```python
from build123d import *

# Parameters (mm, degrees)
SKETCH1_R                = 12.7
BOSS_EXTRUDE1_DEPTH      = 4.7752
SKETCH2_R                = 5.334
BOSS_EXTRUDE2_DEPTH      = 24.13
SKETCH3_R                = 1.27
BOSS_EXTRUDE3_DEPTH      = 2.54
BOSS_EXTRUDE3_DEPTH_BACK = 17.78
SKETCH6_W                = 2.54
SKETCH6_H                = 1.27
BOSS_EXTRUDE4_DEPTH      = 2.54


with BuildPart() as part:
    # Sketch1 → Boss-Extrude1 (new body)
    with BuildSketch(Plane.XY):
        Circle(SKETCH1_R)
    extrude(amount=BOSS_EXTRUDE1_DEPTH)

    # Sketch2 → Boss-Extrude2 (add)
    with BuildSketch(Plane(origin=(0, 0, 0), x_dir=(-1, 0, 0), z_dir=(0, 0, -1))):
        Circle(SKETCH2_R)
    extrude(amount=BOSS_EXTRUDE2_DEPTH)

    # Sketch3 → Boss-Extrude3 (add, two sides)
    with BuildSketch(Plane.XY.offset(4.7752)) as boss_extrude3_sk:
        with Locations((0, 9.525)):
            Circle(SKETCH3_R)
        with Locations((8.248891971, 4.7625)):
            Circle(SKETCH3_R)
        with Locations((8.248891971, -4.7625)):
            Circle(SKETCH3_R)
        with Locations((0, -9.525)):
            Circle(SKETCH3_R)
        with Locations((-8.248891971, -4.7625)):
            Circle(SKETCH3_R)
        with Locations((-8.248891971, 4.7625)):
            Circle(SKETCH3_R)
    extrude(amount=BOSS_EXTRUDE3_DEPTH)
    extrude(boss_extrude3_sk.sketch, amount=-BOSS_EXTRUDE3_DEPTH_BACK)

    # Sketch6 → Boss-Extrude4 (add)
    with BuildSketch(Plane(origin=(0, 0, 0), x_dir=(-1, 0, 0), z_dir=(0, 0, -1))):
        Polygon((1.482073869, 3.837027241), (2.581926131, 3.202027241), (3.851926131, 5.401731767), (2.752073869, 6.036731767), align=None)
        with Locations((5.334, 0)):
            Rectangle(SKETCH6_W, SKETCH6_H)
        Polygon((2.581926131, -3.202027241), (3.851926131, -5.401731767), (2.752073869, -6.036731767), (1.482073869, -3.837027241), align=None)
        Polygon((-1.482073869, -3.837027241), (-2.752073869, -6.036731767), (-3.851926131, -5.401731767), (-2.581926131, -3.202027241), align=None)
        with Locations((-5.334, 0)):
            Rectangle(SKETCH6_W, SKETCH6_H)
        Polygon((-2.581926131, 3.202027241), (-3.851926131, 5.401731767), (-2.752073869, 6.036731767), (-1.482073869, 3.837027241), align=None)
    extrude(amount=BOSS_EXTRUDE4_DEPTH)


solid = part.part
```
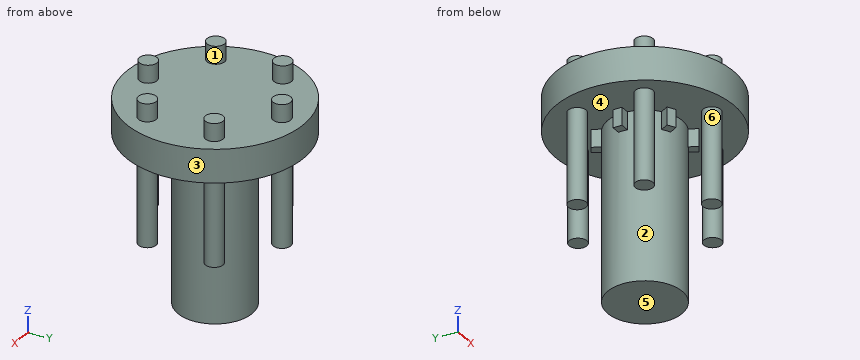
Verification items for the finished model (mm, model axes). Face numbers are marked on the shaded views. A direction names the side the tool comes from. Give positions to 0.01 mm unless a question says otherwise; leave off trailing zeros. Order: outer loops, then holes, each group sorted by start corner. A loop starts at its lowest first (then second) coordinate and runs counter-clockwise, first axis right, second up. Notation, with made-up numbers: (41.25, 22) -> (52.25, 22) arc R28 ccw to (52.25, 61) -> close; hole circle Ø1 at (-35.5, -36.5). An arc over 180 degrees is marked (long way). One line per item, written item: value.
(1) Sectioned sample at B-B on y = 0. Record the cut outline in (x, z), then the cut area to 3 significant figures.
Final values:
outline: (-12.7, 0) -> (-6.6, 0) -> (-6.6, -2.54) -> (-5.33, -2.54) -> (-5.33, -24.13) -> (5.33, -24.13) -> (5.33, -2.54) -> (6.6, -2.54) -> (6.6, 0) -> (12.7, 0) -> (12.7, 4.78) -> (-12.7, 4.78) -> close
area: 385 mm^2
(2) Sectioned sample at D-D on z = 3.5. Record the cut outline in (x, y), then the cut area to 3 significant figures.
Final values:
outline: circle Ø25.4 at (0, 0)
area: 507 mm^2
(3) Scan lines: line 1 along Y through (x, z) = (-0.5, -7); line 2 along Z through (x, y) = (10.25, 3.5); line 3 along Y through (x, z) = (-5.75, -1.5) (3 decimals). Record each from-to range of solid material in increasing order. Write a range as [from, to].
Final values:
line 1: [-10.69, -8.36], [-5.31, 5.31], [8.36, 10.69]
line 2: [0, 4.78]
line 3: [-0.635, 0.635]
(4) Draft check along X on the marked faces 4, 5 and 6. Enter one of: pulls with the +X half, pulls with the -X half, needs draft (parallel to the pull), parting line crosses it, or undercut.
Final values:
face 4: undercut
face 5: needs draft
face 6: parting line crosses it
(5) Gauge pin test, flat ends, axial feed: pin 1 (5 mm diameter, centred on y = 2, z = -21, fed in from -X); pin 2 (2 mm diameter, centred on x = -8, y = -5, fed in from -Z); pin 3 (5 mm diameter, centred on x = 4.5, y = 10, fed in from -Z). Record the tip position at first contact, or that the pin passes through.
Final values:
pin 1: x = -5.33
pin 2: z = -13
pin 3: z = 0
(6) Sectioned sample at C-C on x = 0. Record the cut outline in (y, z) (3 decimals).
Final values:
outline: (-12.7, 0) -> (-10.795, 0) -> (-10.795, -13.005) -> (-8.255, -13.005) -> (-8.255, 0) -> (-5.334, 0) -> (-5.334, -24.13) -> (5.334, -24.13) -> (5.334, 0) -> (8.255, 0) -> (8.255, -13.005) -> (10.795, -13.005) -> (10.795, 0) -> (12.7, 0) -> (12.7, 4.775) -> (10.795, 4.775) -> (10.795, 7.315) -> (8.255, 7.315) -> (8.255, 4.775) -> (-8.255, 4.775) -> (-8.255, 7.315) -> (-10.795, 7.315) -> (-10.795, 4.775) -> (-12.7, 4.775) -> close
(7) Tool access check on the marked faces 1, 2 and 3. Record the directions out of +Z, -Z, +X, -X, +Y, -Y that give a thin tool (end or side, any length) a straight path to the whole face; none if there is none.
Final values:
face 1: +Z
face 2: -Z
face 3: +Z, -Z
(8) Sectioned sample at A-A on z = -12.5. Record the cut outline in (x, y) (1 decimal).
Final values:
outline: circle Ø2.5 at (-8.2, -4.8); circle Ø2.5 at (-8.2, 4.8); circle Ø10.7 at (0, 0); circle Ø2.5 at (0, -9.5); circle Ø2.5 at (0, 9.5); circle Ø2.5 at (8.2, -4.8); circle Ø2.5 at (8.2, 4.8)
